Source: CAD feature listing. Evaluate the final solid. Frame: model axes, mm. A direction names the side the tool comes from. Give positions to 0.01 mm unless a question says otherwise; leave off trailing zeros. Loops run counter-clockwise (first coordinate to the right, second up) from the corner with the lowest first, then second, coordinate; pieces in that order, holes last. Notation, with made-up numbers: M -38.75,26.25 L 20.25,26.25 A23 ccw 20.25,55.25 Z; hole C 16,-31.5 d9. An arc over 180 degrees is marked long. Answer in a Markdown table with one row per item.
```python
from build123d import *

# Parameters (mm, degrees)
SKETCH1_R           = 1.8034
BOSS_EXTRUDE1_DEPTH = 6.35
CHAMFER1_SIZE       = 1.27
CHAMFER1_SIZE2      = 0.340295474


with BuildPart() as part:
    # Sketch1 → Boss-Extrude1 (new body, symmetric)
    with BuildSketch(Plane.XY):
        Circle(SKETCH1_R)
    extrude(amount=BOSS_EXTRUDE1_DEPTH, both=True)

    # Chamfer1
    chamfer1_edges = [part.edges().sort_by_distance(p)[0] for p in [
        (-1.8034, 0, 6.35),
    ]]
    chamfer1_side = [part.faces().sort_by_distance(p)[0] for p in [
        (-1.8034, 0, 0),
    ]]
    chamfer(chamfer1_edges, length=CHAMFER1_SIZE, length2=CHAMFER1_SIZE2, reference=chamfer1_side[0])

    # Sketch2 → Revolve1 (revolve)
    with BuildSketch(Plane(origin=(0, 0, 0), x_dir=(1, 0, 0), z_dir=(0, 1, 0))):
        with BuildLine():
            Line((0, 6.35), (3.175, 6.35))
            Line((3.175, 6.35), (3.175, 7.62))
            ThreePointArc((3.175, 7.62), (2.803025612, 8.518025612), (1.905, 8.89))
            Line((1.905, 8.89), (0, 8.89))
            Line((0, 8.89), (0, 6.35))
        make_face()
    revolve(axis=Axis((0, 0, -6.35), (0, 0, -1)))


solid = part.part
```
1) Pull-direction query (Y, two-part tool) for faces 3 (the flat face through (0, 0, -8.89)), 4 (the conical face through (1.447, 0.456, 6.147)); classes: released by +Y, released by -Y, zero draft, split by the parting line, or undercut.
Reply:
| item | result |
|---|---|
| face 3 | zero draft |
| face 4 | split by the parting line |
2) Pin query (flat end, axial travel): pin 1 Ø2 at (y, z) = (-2, -7.5) entering from -X; pin 2 Ø1 at (x, y) = (0, -2) entering from -Z; pin 3 Ø3 at (x, z) = (2.5, -2.5) entering from +Y. Return the tip coordinate at first contact, or that it passes through.
Reply:
| item | result |
|---|---|
| pin 1 | stops at x = -3.01 |
| pin 2 | stops at z = -8.89 |
| pin 3 | stops at y = 1.5 |
3) Set-up query: faces 1 (the flat face through (-1.4, 1.4, -6.35)), 2 (the cylindrical face through (-0.69, 3.1, -6.99)). Return all of +Z, -Z, +X, -X, +Y, -Y with unobstructed straight access to the full face (end or side cutting, diameter ignored); none if empty.
Reply:
| item | result |
|---|---|
| face 1 | +Z |
| face 2 | +Z, -Z |
4) Section C-C, the plane z = -3.25. Return loops of the section in (x, y).
Reply:
| item | result |
|---|---|
| outline | C 0,0 d3.61 |
5) Material intervals for L1, parallel to Z at x = 0.25, y = 2; L2, parallel to X at y = -0.25, z = -4.75; L3, parallel to X at y = -1.5, z = -2.5, sorted ascending.
Reply:
| item | result |
|---|---|
| L1 | z = -8.89 to -6.35 |
| L2 | x = -1.79 to 1.79 |
| L3 | x = -1 to 1 |
6) Section A-A, the plane y = 0. Return loops of the section in (x, z) (3 decimals), then the cut area to 3 significant figures.
Reply:
| item | result |
|---|---|
| outline | M -3.175,-7.62 A1.27 ccw -1.905,-8.89 L 1.905,-8.89 A1.27 ccw 3.175,-7.62 L 3.175,-6.35 L 1.803,-6.35 L 1.803,5.08 L 1.463,6.35 L -1.463,6.35 L -1.803,5.08 L -1.803,-6.35 L -3.175,-6.35 Z |
| area | 60.8 mm² |
